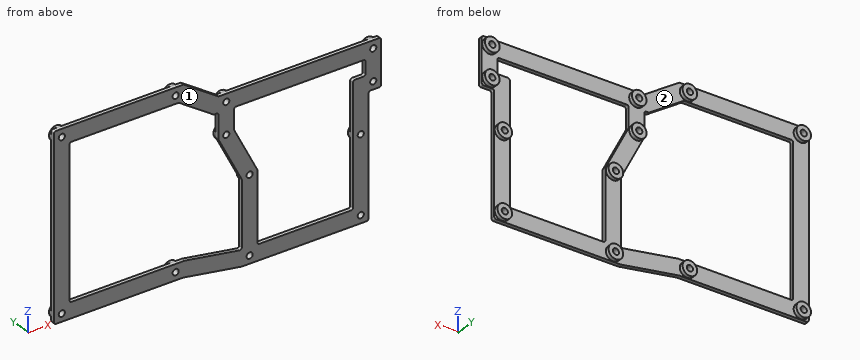
```python
from build123d import *

# Parameters (mm, degrees)
SKETCH1_R           = 1.58
BOSS_EXTRUDE1_DEPTH = 2
SKETCH2_R           = 3.75
SKETCH2_R_2         = 1.58
BOSS_EXTRUDE2_DEPTH = 2
CUT_EXTRUDE5_DEPTH  = 99.635693337
FILLET4_R           = 1


with BuildPart() as part:
    # Sketch1 → Boss-Extrude1 (new body)
    with BuildSketch(Plane(origin=(0, 0, 0), x_dir=(1, 0, 0), z_dir=(0, 1, 0))):
        Polygon((76.6, -14), (83, -14), (83, -38), (-0.5, -38), (-18.5, -50), (-85, -50), (-85, 44), (-18.5, 44), (11.5, 49), (76.6, 49), align=None)
        with Locations(Location((15.5, 45, 0), (0, 0, 270))):
            Circle(SKETCH1_R, mode=Mode.SUBTRACT)
        with Locations(Location((72.6, 45, 0), (0, 0, 270))):
            Circle(SKETCH1_R, mode=Mode.SUBTRACT)
        with Locations(Location((72.6, 5.6, 0), (0, 0, 270))):
            Circle(SKETCH1_R, mode=Mode.SUBTRACT)
        with Locations(Location((15.5, 5.6, 0), (0, 0, 270))):
            Circle(SKETCH1_R, mode=Mode.SUBTRACT)
        with Locations(Location((-81, 40, 0), (0, 0, 270))):
            Circle(SKETCH1_R, mode=Mode.SUBTRACT)
        with Locations(Location((-22.5, 40, 0), (0, 0, 270))):
            Circle(SKETCH1_R, mode=Mode.SUBTRACT)
        with Locations(Location((-22.5, -46, 0), (0, 0, 270))):
            Circle(SKETCH1_R, mode=Mode.SUBTRACT)
        with Locations(Location((-81, -46, 0), (0, 0, 270))):
            Circle(SKETCH1_R, mode=Mode.SUBTRACT)
        with Locations(Location((79, -34, 0), (0, 0, 270))):
            Circle(SKETCH1_R, mode=Mode.SUBTRACT)
        with Locations(Location((79, -18, 0), (0, 0, 270))):
            Circle(SKETCH1_R, mode=Mode.SUBTRACT)
        with Locations(Location((3.5, -34, 0), (0, 0, 270))):
            Circle(SKETCH1_R, mode=Mode.SUBTRACT)
        with Locations(Location((3.5, -18, 0), (0, 0, 270))):
            Circle(SKETCH1_R, mode=Mode.SUBTRACT)
    extrude(amount=BOSS_EXTRUDE1_DEPTH)

    # Sketch2 → Boss-Extrude2 (add)
    # profile 1 of 12: a face of its own
    with BuildSketch(Plane(origin=(0, 2, 0), x_dir=(1, 0, 0), z_dir=(0, 1, 0))):
        with Locations(Location((-81, 40, 0), (0, 0, 90))):
            Circle(SKETCH2_R)
        with Locations(Location((-81, 40, 0), (0, 0, 270))):
            Circle(SKETCH2_R_2, mode=Mode.SUBTRACT)
    # profile 2 of 12: a face of its own
    with BuildSketch(Plane(origin=(0, 2, 0), x_dir=(1, 0, 0), z_dir=(0, 1, 0))):
        with Locations(Location((-22.5, 40, 0), (0, 0, 90))):
            Circle(SKETCH2_R)
        with Locations(Location((-22.5, 40, 0), (0, 0, 270))):
            Circle(SKETCH2_R_2, mode=Mode.SUBTRACT)
    # profile 3 of 12: a face of its own
    with BuildSketch(Plane(origin=(0, 2, 0), x_dir=(1, 0, 0), z_dir=(0, 1, 0))):
        with Locations(Location((-81, -46, 0), (0, 0, 90))):
            Circle(SKETCH2_R)
        with Locations(Location((-81, -46, 0), (0, 0, 270))):
            Circle(SKETCH2_R_2, mode=Mode.SUBTRACT)
    # profile 4 of 12: a face of its own
    with BuildSketch(Plane(origin=(0, 2, 0), x_dir=(1, 0, 0), z_dir=(0, 1, 0))):
        with Locations(Location((-22.5, -46, 0), (0, 0, 90))):
            Circle(SKETCH2_R)
        with Locations(Location((-22.5, -46, 0), (0, 0, 270))):
            Circle(SKETCH2_R_2, mode=Mode.SUBTRACT)
    # profile 5 of 12: a face of its own
    with BuildSketch(Plane(origin=(0, 2, 0), x_dir=(1, 0, 0), z_dir=(0, 1, 0))):
        with Locations(Location((3.5, -34, 0), (0, 0, 90))):
            Circle(SKETCH2_R)
        with Locations(Location((3.5, -34, 0), (0, 0, 270))):
            Circle(SKETCH2_R_2, mode=Mode.SUBTRACT)
    # profile 6 of 12: a face of its own
    with BuildSketch(Plane(origin=(0, 2, 0), x_dir=(1, 0, 0), z_dir=(0, 1, 0))):
        with Locations(Location((3.5, -18, 0), (0, 0, 90))):
            Circle(SKETCH2_R)
        with Locations(Location((3.5, -18, 0), (0, 0, 270))):
            Circle(SKETCH2_R_2, mode=Mode.SUBTRACT)
    # profile 7 of 12: a face of its own
    with BuildSketch(Plane(origin=(0, 2, 0), x_dir=(1, 0, 0), z_dir=(0, 1, 0))):
        with Locations(Location((15.5, 5.6, 0), (0, 0, 90))):
            Circle(SKETCH2_R)
        with Locations(Location((15.5, 5.6, 0), (0, 0, 270))):
            Circle(SKETCH2_R_2, mode=Mode.SUBTRACT)
    # profile 8 of 12: a face of its own
    with BuildSketch(Plane(origin=(0, 2, 0), x_dir=(1, 0, 0), z_dir=(0, 1, 0))):
        with Locations(Location((72.6, 5.6, 0), (0, 0, 90))):
            Circle(SKETCH2_R)
        with Locations(Location((72.6, 5.6, 0), (0, 0, 270))):
            Circle(SKETCH2_R_2, mode=Mode.SUBTRACT)
    # profile 9 of 12: a face of its own
    with BuildSketch(Plane(origin=(0, 2, 0), x_dir=(1, 0, 0), z_dir=(0, 1, 0))):
        with Locations(Location((79, -18, 0), (0, 0, 90))):
            Circle(SKETCH2_R)
        with Locations(Location((79, -18, 0), (0, 0, 270))):
            Circle(SKETCH2_R_2, mode=Mode.SUBTRACT)
    # profile 10 of 12: a face of its own
    with BuildSketch(Plane(origin=(0, 2, 0), x_dir=(1, 0, 0), z_dir=(0, 1, 0))):
        with Locations(Location((79, -34, 0), (0, 0, 90))):
            Circle(SKETCH2_R)
        with Locations(Location((79, -34, 0), (0, 0, 270))):
            Circle(SKETCH2_R_2, mode=Mode.SUBTRACT)
    # profile 11 of 12: a face of its own
    with BuildSketch(Plane(origin=(0, 2, 0), x_dir=(1, 0, 0), z_dir=(0, 1, 0))):
        with Locations(Location((72.6, 45, 0), (0, 0, 90))):
            Circle(SKETCH2_R)
        with Locations(Location((72.6, 45, 0), (0, 0, 270))):
            Circle(SKETCH2_R_2, mode=Mode.SUBTRACT)
    # profile 12 of 12: a face of its own
    with BuildSketch(Plane(origin=(0, 2, 0), x_dir=(1, 0, 0), z_dir=(0, 1, 0))):
        with Locations(Location((15.5, 45, 0), (0, 0, 90))):
            Circle(SKETCH2_R)
        with Locations(Location((15.5, 45, 0), (0, 0, 270))):
            Circle(SKETCH2_R_2, mode=Mode.SUBTRACT)
    extrude(amount=BOSS_EXTRUDE2_DEPTH)

    # Sketch7 → Cut-Extrude5 (cut, through all)
    with BuildSketch(Plane(origin=(0, 2, 0), x_dir=(1, 0, 0), z_dir=(0, 1, 0))):
        Polygon((-0.5, -17.04145027), (11.5, 6.55854973), (11.5, 40.88964996), (-17.837899758, 36), (-77, 36), (-77, -42), (-20.922205102, -42), (-2.922205102, -30), (-0.5, -30), align=None)
        Polygon((19.5, 4.64145027), (19.5, 41), (68.6, 41), (68.6, -22), (75, -22), (75, -30), (7.5, -30), (7.5, -18.95854973), align=None)
    extrude(amount=-CUT_EXTRUDE5_DEPTH, mode=Mode.SUBTRACT)

    # Fillet4
    fillet4_edges = [part.edges().sort_by_distance(p)[0] for p in [
        (7.5, 1, 18.95854973),
        (19.5, 1, -4.64145027),
        (19.5, 1, -41),
        (68.6, 1, -41),
        (68.6, 1, 22),
        (75, 1, 22),
        (75, 1, 30),
        (7.5, 1, 30),
        (-18.5, 1, -44),
        (11.5, 1, -49),
        (76.6, 1, -49),
        (76.6, 1, 14),
        (83, 1, 14),
        (83, 1, 38),
        (-0.5, 1, 38),
        (-17.837899758, 1, -36),
        (11.5, 1, -40.88964996),
        (-18.5, 1, 50),
        (11.5, 1, -6.55854973),
        (-0.5, 1, 17.04145027),
        (-0.5, 1, 30),
        (-85, 1, 50),
        (-2.922205102, 1, 30),
        (-20.922205102, 1, 42),
        (-85, 1, -44),
        (-77, 1, 42),
        (-77, 1, -36),
    ]]
    fillet(fillet4_edges, radius=FILLET4_R)


solid = part.part
```
Geometry: final body of the model. Coordinates: model frame, mm. Face numbers are marked on the shaded views. Give positions to 0.01 mm unless a question says otherwise; leave off trailing zeros. Loops run counter-clockwise (first coordinate to the right, second up) from the corner with the lowest first, then second, coordinate; pieces in that order, holes last. Notation, with made-up numbers: (3, 2) -> (37, 2) arc R28 cw to (37, 28) -> close; hole circle Ø11 at (-13.5, -17.75). An arc over 180 degrees is marked (long way). Return JSON: item names as keys, results as strings.
Item 1: Section A-A, the plane y = 2.85. Count the separate pieces of the cut face and the enclosed holes in it, plus the area to 3 significant figures.
Filled in:
{"separate pieces": "12", "enclosed holes": "12", "area": "436 mm^2"}
Item 2: Pin query (flat end, axial travel): P1, Ø1, axis at x = 7, z = 0, coming from the -Y side; P2, Ø12, axis at x = 11.5, z = -25, coming from the +Y side; P3, Ø0.6, axis at x = 73, y = 1, coming from the +Z side; P4, Ø1.5, axis at y = 2.5, z = -11.5, coming from the +X side. Return the tip coordinate at first contact, or that it passes through.
Filled in:
{"P1": "through", "P2": "y = 2", "P3": "z = 38", "P4": "x = 76.6"}
Item 3: Mould query, pull axis X, two halves, no side actions, for the marked faces 1 and 2. Classes: released by +X, released by -X, zero draft, split by the parting line, or undercut.
Filled in:
{"face 1": "zero draft", "face 2": "undercut"}
Item 4: Section D-D, the plane z = -22.5. Output: boundary loops of the cut face in (x, y), plus the area to 3 significant figures.
Filled in:
{"outline": "(-85, 0) -> (-77, 0) -> (-77, 2) -> (-85, 2) -> close; (11.5, 0) -> (19.5, 0) -> (19.5, 2) -> (11.5, 2) -> close; (68.6, 0) -> (76.6, 0) -> (76.6, 2) -> (68.6, 2) -> close", "area": "48.0 mm^2"}
Item 5: Section B-B, the plane x = -81. Output: boundary loops of the cut face in (y, z), plus the area to 3 significant figures.
Filled in:
{"outline": "(0, -44) -> (2, -44) -> (2, -43.75) -> (4, -43.75) -> (4, -41.58) -> (0, -41.58) -> close; (0, -38.42) -> (4, -38.42) -> (4, -36.25) -> (2, -36.25) -> (2, 42.25) -> (4, 42.25) -> (4, 44.42) -> (0, 44.42) -> close; (0, 47.58) -> (4, 47.58) -> (4, 49.75) -> (2, 49.75) -> (2, 50) -> (0, 50) -> close", "area": "193 mm^2"}
Item 6: Line query: line 1 (Z direction, x = 72.6, y = 1.5); line 2 (X direction, y = 2.5, z = -45); line 3 (X direction, y = 3.8, z = 33). Output: solid intervals per line, ascending.
Filled in:
{"line 1": "-49 to -46.58, -43.42 to -7.18, -4.02 to 22, 30 to 38", "line 2": "11.75 to 13.92, 17.08 to 19.25, 68.85 to 71.02, 74.18 to 76.35", "line 3": "-0.11 to 2.28, 4.72 to 7.11, 75.39 to 77.78, 80.22 to 82.61"}
Item 7: Section C-C, the plane x = 58. Output: boundary loops of the cut face in (y, z).
Filled in:
{"outline": "(0, -49) -> (2, -49) -> (2, -41) -> (0, -41) -> close; (0, 30) -> (2, 30) -> (2, 38) -> (0, 38) -> close"}
